For this review, take the finished solid that the model builds, in its own axes (mm). A direction names the side the tool comes from. Give positions to 0.01 mm unless a question says otherwise; leave off trailing zeros. Order: outer loops, then holes, each group sorted by start corner. A loop starts at its lowest first (then second) coordinate and runs counter-clockwise, first axis right, second up.
from build123d import *


with BuildPart() as f1:
    # F0 (on Front) → F1 (revolve)
    with BuildSketch(Plane.XZ):
        Polygon((-4.7625, 0.631558), (-4.7625, 1.826994), (-7.1625, 1.826994), (-7.1625, -6.801847), (0, -6.801847), (0, -4.7625), (-4.7625, -4.7625), align=None)
        with BuildLine():
            Line((-4.398125, 1.826994), (-4.7625, 1.826994))
            Line((-4.7625, 1.826994), (-4.7625, 0.631558))
            Line((-4.7625, 0.631558), (-4.720439, 0.631558))
            ThreePointArc((-4.720439, 0.631558), (-4.598295, 1.239794), (-4.398125, 1.826994))
        make_face()
    revolve(axis=Axis((0, 0, -5.782173), (0, 0, 1)))


solid = f1.part
1) To check wall thickness, follow line 1 (Y direction, x = 0, z = -2.3); line 2 (Z direction, x = -2, y = 2.25). State the ranges of each line that lie inside material, in increasing order.
Answer sheet:
line 1: y = -7.16 to -4.76, 4.76 to 7.16
line 2: z = -6.8 to -4.76
2) Tool access review of faces 1 (the face through (0, 0, -6.802)), 2 (the face through (3.78, 2.9, -2.03)): name each direction out of +Z, -Z, +X, -X, +Y, -Y from which nothing blocks a thin tool from reaching the whole face with its end or side.
Answer sheet:
face 1: -Z, +X, -X, +Y, -Y
face 2: none
3) Clearance check with flat-ended pins moving along their axes: pin 1 (4 mm diameter, centred on x = -5.5, z = -4, fed in from +Y); pin 2 (7.5 mm diameter, centred on x = 0, y = 0, fed in from +Z); pin 3 (4 mm diameter, centred on y = -3, z = -4, fed in from -X). State where each tip first meets the part, or that it passes through.
Answer sheet:
pin 1: stops at y = 6.25
pin 2: stops at z = -4.76
pin 3: stops at x = -7.09
4) We need section B-B on y = 6. Give the boundary of the cut face in (x, z).
Answer sheet:
outline: (-3.91, -6.8) - (3.91, -6.8) - (3.91, 1.83) - (-3.91, 1.83) - close
5) We need section A-A on z = -3.75. Give the boundary of the cut face in (x, y) (1 decimal).
Answer sheet:
outline: circle Ø14.3 at (0, 0); hole circle Ø9.5 at (0, 0)
6) Draft analysis for pull direction Y (two halves, no side actions). For faces 3 (the face through (-6.832, -2.151, -2.548)), 4 (the face through (0, 5, 1.827)), 5 (the face through (0, 0, -4.762)), state which applies: +Y half, -Y half, draft (parallel to the pull), parting line (faces both ways), or undercut.
Answer sheet:
face 3: parting line
face 4: draft
face 5: undercut
